```python
from build123d import *

# Parameters (mm, degrees)
SKETCH1_W           = 60
SKETCH1_H           = 48
SKETCH1_R           = 1.32
BOSS_EXTRUDE1_DEPTH = 6
SKETCH2_R           = 3.25
CUT_EXTRUDE1_DEPTH  = 4


with BuildPart() as part:
    # Sketch1 → Boss-Extrude1 (new body)
    with BuildSketch(Plane.XY):
        Rectangle(SKETCH1_W, SKETCH1_H)
        with Locations((0, -15.875)):
            Circle(SKETCH1_R, mode=Mode.SUBTRACT)
        with Locations((-15.875, 0)):
            Circle(SKETCH1_R, mode=Mode.SUBTRACT)
        with Locations((0, 15.875)):
            Circle(SKETCH1_R, mode=Mode.SUBTRACT)
        with Locations((15.875, 0)):
            Circle(SKETCH1_R, mode=Mode.SUBTRACT)
        with Locations((-25, 20)):
            Circle(SKETCH1_R, mode=Mode.SUBTRACT)
        with Locations((25, 20)):
            Circle(SKETCH1_R, mode=Mode.SUBTRACT)
        with Locations((25, -20)):
            Circle(SKETCH1_R, mode=Mode.SUBTRACT)
        with Locations((-25, -20)):
            Circle(SKETCH1_R, mode=Mode.SUBTRACT)
    extrude(amount=BOSS_EXTRUDE1_DEPTH)

    # Sketch2 → Cut-Extrude1 (cut)
    with BuildSketch(Plane(origin=(0, 0, 0), x_dir=(-1, 0, 0), z_dir=(0, 0, -1))):
        with Locations((0, 15.875)):
            Circle(SKETCH2_R)
        with Locations((15.875, 0)):
            Circle(SKETCH2_R)
        with Locations((0, -15.875)):
            Circle(SKETCH2_R)
        with Locations((-15.875, 0)):
            Circle(SKETCH2_R)
    extrude(amount=-CUT_EXTRUDE1_DEPTH, mode=Mode.SUBTRACT)


solid = part.part
```
The model under review builds one solid part; all positions refer to its coordinate system, in mm. A direction names the side the tool comes from. Round coordinates to 2 decimals unless told otherwise and drop trailing zeros. Write each loop counter-clockwise with the first axis right and the second up, starting at its lowest first coordinate (ties: lowest second). Pieces come first, ordered by that corner, then holes. Notation, with made-up numbers: (45, -32.5) - (50, -32.5) arc R9 ccw to (50, -19.5) - close; hole circle Ø4 at (27.25, 14.25). An arc over 180 degrees is marked (long way). Answer as CSV lines item,"result". Start each with the question number.
(1) We need section A-A on x = 25. State the section outline as (y, z) points, plus the area to 3 significant figures.
(2) Draft analysis for pull direction X (two halves, no side actions). For faces 3 (the cylindrical face through (-0.286, 14.586, 4.986)), 4 (the flat face through (30, 0, 3)), 5 (the flat face through (0, 0, 6)), state which applies: pulls with the +X half, pulls with the -X half, needs draft (parallel to the pull), parting line crosses it, or undercut.
(3) To check wall thickness, follow line 1 (Y direction, x = 0, z = 2.55) (3 decimals); line 2 (Y direction, x = -25, z = 3.1); line 3 (X direction, y = -0.5, z = 5.6). State the ranges of each line that lie inside material, in increasing order.
(4) For pin 1 Ø3 at (x, y) = (-16.5, -0.5) entering from -Z, flat-tipped, find the tip position at first contact; note if it passes through.
(5) We need section C-C on z = 3.25. Give the number of separate pieces and of enclosed holes in the cut face, plus the area to 3 significant figures.
(6) We need section D-D on x = 0. State the section outline as (y, z) points (3 decimals).
(7) For faces 1 (the cylindrical face through (0.423, -12.653, 1.972)), 2 (the flat face through (0, -24, 3)), list the 3-axis set-ups (+Z, -Z, +X, -X, +Y, -Y) from which the entire face can be reached by the end or side of a thin tool; tool diameter is ignored.
(8) We need section B-B on y = -20. State the section outline as (x, z) points.
Worked answers:
1,outline,"(-24, 0) - (-21.32, 0) - (-21.32, 6) - (-24, 6) - close; (-18.68, 0) - (18.68, 0) - (18.68, 6) - (-18.68, 6) - close; (21.32, 0) - (24, 0) - (24, 6) - (21.32, 6) - close"
1,area,"256 mm²"
2,face 3,"undercut"
2,face 4,"pulls with the +X half"
2,face 5,"needs draft"
3,line 1,"-24 to -19.125, -12.625 to 12.625, 19.125 to 24"
3,line 2,"-24 to -21.32, -18.68 to 18.68, 21.32 to 24"
3,line 3,"-30 to -17.1, -14.65 to 14.65, 17.1 to 30"
4,pin 1,"z = 4"
5,separate pieces,"1"
5,enclosed holes,"8"
5,area,"2,730 mm²"
6,outline,"(-24, 0) - (-19.125, 0) - (-19.125, 4) - (-17.195, 4) - (-17.195, 6) - (-24, 6) - close; (-14.555, 4) - (-12.625, 4) - (-12.625, 0) - (12.625, 0) - (12.625, 4) - (14.555, 4) - (14.555, 6) - (-14.555, 6) - close; (17.195, 4) - (19.125, 4) - (19.125, 0) - (24, 0) - (24, 6) - (17.195, 6) - close"
7,face 1,"-Z"
7,face 2,"+Z, -Z, +X, -X, -Y"
8,outline,"(-30, 0) - (-26.32, 0) - (-26.32, 6) - (-30, 6) - close; (-23.68, 0) - (23.68, 0) - (23.68, 6) - (-23.68, 6) - close; (26.32, 0) - (30, 0) - (30, 6) - (26.32, 6) - close"
